Geometry check sheet. Reference: the model listing, model coordinates, mm. A direction names the side the tool comes from. Round coordinates to 2 decimals unless told otherwise and drop trailing zeros. Write each loop counter-clockwise with the first axis right and the second up, starting at its lowest first coordinate (ties: lowest second). Pieces come first, ordered by that corner, then holes. Notation, with made-up numbers: (3, 0) -> (59, 0) arc R30 ccw to (59, 31) -> close; hole circle Ø9 at (-5, 33.25). An arc over 180 degrees is marked (long way). Use a Markdown table: item, result.
```python
from build123d import *

# Parameters (mm, degrees)
CROQUIS1_W              = 80
CROQUIS1_H              = 60
SALIENTE_EXTRUIR1_DEPTH = 10
CROQUIS2_W              = 70
CROQUIS2_H              = 40
SALIENTE_EXTRUIR2_DEPTH = 10
CROQUIS3_R              = 6
SALIENTE_EXTRUIR3_DEPTH = 10


with BuildPart() as part:
    # Croquis1 → Saliente-Extruir1 (new body)
    with BuildSketch(Plane.XY):
        Rectangle(CROQUIS1_W, CROQUIS1_H)
    extrude(amount=SALIENTE_EXTRUIR1_DEPTH)

    # Croquis2 → Saliente-Extruir2 (add)
    with BuildSketch(Plane.XY.offset(10)):
        with Locations((35, 0)):
            Rectangle(CROQUIS2_W, CROQUIS2_H)
    extrude(amount=SALIENTE_EXTRUIR2_DEPTH)

    # Croquis3 → Saliente-Extruir3 (add)
    with BuildSketch(Plane.XY.offset(20)):
        with Locations((55, 0)):
            Circle(CROQUIS3_R)
    extrude(amount=SALIENTE_EXTRUIR3_DEPTH)


solid = part.part
```
(1) Gauge pin test, flat ends, axial feed: pin 1 Ø4 at (x, y) = (37.5, 4) entering from -Z; pin 2 Ø5 at (y, z) = (-4, 14.5) entering from -X; pin 3 Ø20 at (x, y) = (38.5, -6) entering from +Z; pin 4 Ø5 at (x, z) = (31, 16) entering from -Y. Record the tip position at first contact, or that the pin passes through.
A:
| item | result |
|---|---|
| pin 1 | stops at z = 0 |
| pin 2 | stops at x = 0 |
| pin 3 | stops at z = 20 |
| pin 4 | stops at y = -20 |
(2) Section check A-A on x = 55. Record the cut outline in (y, z), plus the area to 3 significant figures.
A:
| item | result |
|---|---|
| outline | (-20, 10) -> (20, 10) -> (20, 20) -> (6, 20) -> (6, 30) -> (-6, 30) -> (-6, 20) -> (-20, 20) -> close |
| area | 520 mm2 |
(3) Section check C-C on z = 6.5. Record the cut outline in (x, y).
A:
| item | result |
|---|---|
| outline | (-40, -30) -> (40, -30) -> (40, 30) -> (-40, 30) -> close |
(4) Access from +Z, -Z, +X, -X, +Y, -Y to the whole of each face (thin tool, end or side, straight path). Record for faces 1 (the face through (40, 0, 5)), 2 (the face through (35, 20, 15)), 3 (the face through (35, -20, 15)), 4 (the face through (49, 0, 25)), 5 (the face through (0, 0, 15)).
A:
| item | result |
|---|---|
| face 1 | -Z, +X, +Y, -Y |
| face 2 | +Z, +X, -X, +Y |
| face 3 | +Z, +X, -X, -Y |
| face 4 | +Z |
| face 5 | +Z, -X, +Y, -Y |
(5) Section check B-B on y = 7.5. Record the cut outline in (x, z), plus the area to 3 significant figures.
A:
| item | result |
|---|---|
| outline | (-40, 0) -> (40, 0) -> (40, 10) -> (70, 10) -> (70, 20) -> (0, 20) -> (0, 10) -> (-40, 10) -> close |
| area | 1,500 mm2 |
(6) Section check D-D on y = 0. Record the cut outline in (x, z), plus the area to 3 significant figures.
A:
| item | result |
|---|---|
| outline | (-40, 0) -> (40, 0) -> (40, 10) -> (70, 10) -> (70, 20) -> (61, 20) -> (61, 30) -> (49, 30) -> (49, 20) -> (0, 20) -> (0, 10) -> (-40, 10) -> close |
| area | 1,620 mm2 |
(7) Thickness scan on line 1 (Z direction, x = -10.5, y = 7.5); line 2 (Z direction, x = 41, y = 16); line 3 (Y direction, x = 40, z = 18). Record the ranges inside material, lowest first.
A:
| item | result |
|---|---|
| line 1 | z = 0 to 10 |
| line 2 | z = 10 to 20 |
| line 3 | y = -20 to 20 |
